The listing builds one solid part. Answer for the finished solid, in the listing's coordinates (mm). A direction names the side the tool comes from. Coordinates: 2 decimals unless noted, no trailing zeros. Loops run counter-clockwise (first coordinate to the right, second up) from the corner with the lowest first, then second, coordinate; pieces in that order, holes last. Notation, with made-up numbers: (75.25, 37.5) - (126.25, 37.5) arc R33 cw to (126.25, 76.5) - close; hole circle Ø6 at (46, 23.25). An arc over 180 degrees is marked (long way). Return JSON: item names as keys, results as strings. Group by question number.
1. Which of the six approach directions +Z, -Z, +X, -X, +Y, -Y give full straight-line access (tool end or side, diameter ignored) to faces 4 (the face through (-22.4, -4.3, 37)), 5 (the face through (-27.475, 1.181, 16.269)), 6 (the face through (25, -2, 18))?
2. Section B-B (z = 13) is taken. Write down the section's boundary in (x, y), and give its area (3 significant figures).
3. Section A-A (y = 0) is taken. Write down the section's boundary in (x, z).
4. Each of these flat-tipped pins is pushed along its axis until it touches: P1, Ø2, axis at x = -23.5, z = 10, coming from the +Y side; P2, Ø4, axis at y = -10, z = 31.5, coming from the -X side; P3, Ø3, axis at x = -5.5, z = 3.5, coming from the -Y side; P4, Ø18, axis at x = 13, y = -1, coming from the -Z side. Where does it stop, or does it pass through?
5. The mould has two halves that part along Y. Classify faces 1 (the face through (-10.3, -20.2, 0)), 2 (the face through (-22.48, -0.96, 18.24)), 3 (the face through (-29.972, 1.291, 35.986)): pulls with the +Y half, pulls with the -Y half, needs draft (parallel to the pull), parting line crosses it, or undercut.
6. Find the intervals of material crossed by line 1 along Y through (x, z) = (0, 20); line 2 along Y through (x, z) = (1.5, 13); line 3 along X through (y, z) = (17, 17), in increasing order.
```python
from build123d import *

# Parameters (mm, degrees)
EXTRUDE_1_DEPTH = 35
EXTRUDE_2_DEPTH = 2
FILLET_1_R      = 2


with BuildPart() as part:
    # Эскиз1 → Бобышка-Вытянуть1 (new body)
    with BuildSketch(Plane.XY):
        with BuildLine():
            Line((22.410934831, 2), (27.427176304, 2))
            ThreePointArc((27.427176304, 2), (-27.5, 0), (27.427176304, -2))
            Line((27.427176304, -2), (22.410934831, -2))
            ThreePointArc((22.410934831, -2), (-22.5, 0), (22.410934831, 2))
        make_face()
    extrude(amount=EXTRUDE_1_DEPTH)

    # Эскиз2 → Бобышка-Вытянуть2 (add)
    with BuildSketch(Plane.XY.offset(35)):
        with BuildLine():
            Line((22.410934831, 2), (29.933259094, 2))
            ThreePointArc((29.933259094, 2), (-30, 0), (29.933259094, -2))
            Line((29.933259094, -2), (22.410934831, -2))
            ThreePointArc((22.410934831, -2), (-22.5, 0), (22.410934831, 2))
        make_face()
    extrude(amount=EXTRUDE_2_DEPTH)

    # Скругление1
    fillet_1_edges = [part.edges().sort_by_distance(p)[0] for p in [
        (-27.5, 0, 35),
    ]]
    fillet(fillet_1_edges, radius=FILLET_1_R)


solid = part.part
```
The answers:
{
 "1": {"face 4": "+Z, +X, -X, +Y, -Y", "face 5": "-Z", "face 6": "+Z, -Z, +X"},
 "2": {"outline": "(22.41, -2) arc R22.5 cw (long way) to (22.41, 2) - (27.43, 2) arc R27.5 ccw (long way) to (27.43, -2) - close", "area": "765 mm2"},
 "3": {"outline": "(-30, 35) - (-29.5, 35) arc R2 cw to (-27.5, 33) - (-27.5, 0) - (-22.5, 0) - (-22.5, 37) - (-30, 37) - close"},
 "4": {"P1": "stops at y = 15.81", "P2": "stops at x = -26.31", "P3": "stops at y = -27.21", "P4": "passes through"},
 "5": {"face 1": "needs draft", "face 2": "undercut", "face 3": "parting line crosses it"},
 "6": {"line 1": "y = -27.5 to -22.5, 22.5 to 27.5", "line 2": "y = -27.46 to -22.45, 22.45 to 27.46", "line 3": "x = -21.62 to -14.74, 14.74 to 21.62"}
}
